The listing builds one solid part. Answer for the finished solid, in the listing's coordinates (mm). Face numbers are marked on the shaded views. Coordinates: 2 decimals unless noted, no trailing zeros. Order: outer loops, then holes, each group sorted by start corner. A loop starts at its lowest first (then second) coordinate and runs counter-clockwise, first axis right, second up. Notation, with made-up numbers: (-36, -33) -> (-11, -33) arc R20 ccw to (-11, -28) -> close; hole circle Ø9 at (10.25, 73.5). An arc over 180 degrees is marked (long way). Return JSON: item names as keys, results as strings.
```python
from build123d import *

# Parameters (mm, degrees)
SKETCH003_W   = 10
SKETCH003_H   = 10
PAD003_DEPTH  = 2
SKETCH001_W   = 30
SKETCH001_H   = 50
SKETCH001_W_2 = 10
SKETCH001_H_2 = 30
PAD001_DEPTH  = 2
PAD002_DEPTH  = 2
PAD_DEPTH     = 2
SKETCH004_W   = 190
SKETCH004_H   = 90
PAD004_DEPTH  = 4
SKETCH005_W   = 170
SKETCH005_H   = 70
POCKET_DEPTH  = 2


with BuildPart() as obj1:
    # Sketch003 → Pad003 (new body)
    with BuildSketch(Plane(origin=(40, 0, 0), x_dir=(1, 0, 0), z_dir=(0, 0, 1))):
        Polygon((0, 0), (0, 50), (30, 50), (30, 0), (20, 0), (20, 20), (10, 20), (10, 0), align=None)
        with Locations((15.098105, 34.798059)):
            Rectangle(SKETCH003_W, SKETCH003_H, mode=Mode.SUBTRACT)
    extrude(amount=PAD003_DEPTH)


with BuildPart() as obj2:
    # Sketch001 → Pad001 (new body)
    with BuildSketch(Plane(origin=(-40, 0, 0), x_dir=(1, 0, 0), z_dir=(0, 0, 1))):
        with Locations((15, 25)):
            Rectangle(SKETCH001_W, SKETCH001_H)
        with Locations((15, 25)):
            Rectangle(SKETCH001_W_2, SKETCH001_H_2, mode=Mode.SUBTRACT)
    extrude(amount=PAD001_DEPTH)


with BuildPart() as obj3:
    # Sketch002 → Pad002 (new body)
    with BuildSketch(Plane.XY):
        Polygon((0, 50), (0, 0), (30, 0), (30, 10), (10, 10), (10, 50), align=None)
    extrude(amount=PAD002_DEPTH)


with BuildPart() as hola:
    # Sketch → Pad (new body)
    with BuildSketch(Plane(origin=(-80, 0, 0), x_dir=(1, 0, 0), z_dir=(0, 0, 1))):
        Polygon((0, 0), (10, 0), (10, 20), (20, 20), (20, 0), (30, 0), (30, 50), (20, 50), (20, 30), (10, 30), (10, 50), (0, 50), align=None)
    extrude(amount=PAD_DEPTH)

    # Fusion: union obj1, obj2, obj3
    add(obj1.part)
    add(obj2.part)
    add(obj3.part)


with BuildPart() as hola_1:
    # Fusion placement: moved
    add(hola.part.moved(Location((0, 0, 2))))


with BuildPart() as fusion001:
    # Sketch004 → Pad004 (new body)
    with BuildSketch(Plane.XY):
        with Locations((-4.907433, 24.638643)):
            Rectangle(SKETCH004_W, SKETCH004_H)
    extrude(amount=PAD004_DEPTH)

    # Sketch005 → Pocket (cut)
    with BuildSketch(Plane.XY.offset(4)):
        with Locations((-4.929122, 25.012712)):
            Rectangle(SKETCH005_W, SKETCH005_H)
    extrude(amount=-POCKET_DEPTH, mode=Mode.SUBTRACT)

    # Fusion001: union HOLA
    add(hola_1.part)


solid = fusion001.part
```
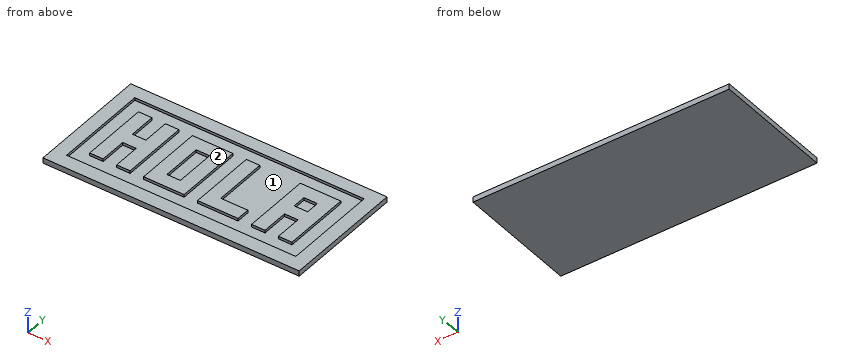
Item 1: Find the intervals of material crossed by probe 1 along Y at (x, z) = (-19.5, 3.5); probe 2 along Y at (x, z) = (-28, 3.8); probe 3 along Y at (x, z) = (71.5, 3.55), in increasing order.
Answer list:
{"probe 1": "-20.36 to -9.99, 0 to 50, 60.01 to 69.64", "probe 2": "-20.36 to -9.99, 0 to 10, 40 to 50, 60.01 to 69.64", "probe 3": "-20.36 to -9.99, 60.01 to 69.64"}
Item 2: Determine the mould class of the marked faces 1 and 2 for opening direction X: pulls with the +X half, pulls with the -X half, needs draft (parallel to the pull), parting line crosses it, or undercut.
Answer list:
{"face 1": "undercut", "face 2": "needs draft"}
Item 3: The part is cut by section A-A on x = -44. Determine the outline of the cut face in (y, z).
Answer list:
{"outline": "(-20.36, 0) -> (69.64, 0) -> (69.64, 4) -> (60.01, 4) -> (60.01, 2) -> (-9.99, 2) -> (-9.99, 4) -> (-20.36, 4) -> close"}
Item 4: The part is cut by section B-B on y = 44.5. Determine the outline of the cut face in (x, z), plus the area to 3 significant figures.
Answer list:
{"outline": "(-99.91, 0) -> (90.09, 0) -> (90.09, 4) -> (80.07, 4) -> (80.07, 2) -> (70, 2) -> (70, 4) -> (40, 4) -> (40, 2) -> (10, 2) -> (10, 4) -> (0, 4) -> (0, 2) -> (-10, 2) -> (-10, 4) -> (-40, 4) -> (-40, 2) -> (-50, 2) -> (-50, 4) -> (-60, 4) -> (-60, 2) -> (-70, 2) -> (-70, 4) -> (-80, 4) -> (-80, 2) -> (-89.93, 2) -> (-89.93, 4) -> (-99.91, 4) -> close", "area": "600 mm2"}
Item 5: The part is cut by section C-C on z = 2.6. Count the separate pieces of the cut face and the enclosed holes in it, plus the area to 3 significant figures.
Answer list:
{"separate pieces": "5", "enclosed holes": "3", "area": "9,400 mm2"}
Item 6: The part is cut by section D-D on x = -64. Determine the outline of the cut face in (y, z).
Answer list:
{"outline": "(-20.36, 0) -> (69.64, 0) -> (69.64, 4) -> (60.01, 4) -> (60.01, 2) -> (30, 2) -> (30, 4) -> (20, 4) -> (20, 2) -> (-9.99, 2) -> (-9.99, 4) -> (-20.36, 4) -> close"}
